For this review, take the finished solid that the model builds, in its own axes (mm). A direction names the side the tool comes from. Coordinates: 2 decimals unless noted, no trailing zeros. Loops run counter-clockwise (first coordinate to the right, second up) from the corner with the lowest first, then second, coordinate; pieces in that order, holes last. Notation, with made-up numbers: M -37.5,62 L 10.5,62 A28 ccw 10.5,88 Z; hole C 11.5,-14.75 d2. An arc over 180 degrees is marked long. Answer as a JSON object with one key per item and string values. Group by question number.
Item 1: Add section B-B (y = 13). State the section outline as (x, z) points, then the cut area to 3 significant figures.
Item 2: Wall thickness on L1, parallel to Y at x = 2, z = -13; L2, parallel to Y at x = -6.5, z = -2.5; L3, parallel to Z at x = 19, y = 13: over which ranges is each line inside the solid? List them lowest first. Write a range as from..to.
Item 3: Mouldability with a two-part tool opening along Z and no side actions: class faces 4 (the face through (1, 0, 0)), 5 (the face through (1, 20, -8)), 6 (the face through (1, 11, -12)) as +Z half, -Z half, draft (parallel to the pull), parting line (faces both ways), or undercut.
Item 4: Add section D-D (y = 0). State the section outline as (x, z) points.
Item 5: Add section C-C (z = -8.75). State the section outline as (x, y) points, then the cut area to 3 significant figures.
Item 6: Insertion check: pin 1 (9 mm diameter, centred on x = 35, y = 0, fed in from -Z); pin 2 (2 mm diameter, centred on y = 11, z = -10.5, fed in from -X). Each pin has a flat end and moves straight along its axis. Give the tip position at first contact, or say it passes through.
Item 7: Tool access review of faces 1 (the face through (1, 15, -15)), 2 (the face through (1, -14, -14)), 3 (the face through (1, 10, -12)): name each direction out of +Z, -Z, +X, -X, +Y, -Y from which nothing blocks a thin tool from reaching the whole face with its end or side.
from build123d import *

# Parameters (mm, degrees)
F1_DEPTH = 52
F2_R     = 4
F3_DEPTH = 12.5
F4_R     = 1
F5_R     = 1
F6_R     = 1


with BuildPart() as f1:
    # F0 (on Right) → F1 (new body, symmetric)
    with BuildSketch(Plane.YZ):
        Polygon((20, 0), (-20, 0), (-20, -15), (-10, -15), (-10, -11), (-11, -11), (-11, -14), (-19, -14), (-19, -1), (19, -1), (19, -14), (11, -14), (11, -11), (10, -11), (10, -15), (20, -15), align=None)
    extrude(amount=F1_DEPTH, both=True)

    # F2 (on Top) → F3 (cut, symmetric)
    with BuildSketch(Plane.XY):
        with Locations((-35, 0)):
            Circle(F2_R)
        with Locations((35, 0)):
            Circle(F2_R)
    extrude(amount=F3_DEPTH, both=True, mode=Mode.SUBTRACT)

    # F4
    f4_edges = [f1.edges().sort_by_distance(p)[0] for p in [
        (0, -20, -15),
        (0, -20, 0),
        (0, -10, -15),
        (0, 10, -15),
        (0, 20, -15),
        (0, 20, 0),
        (0, 19, -14),
        (0, -19, -14),
    ]]
    fillet(f4_edges, radius=F4_R)

    # F5
    f5_edges = [f1.edges().sort_by_distance(p)[0] for p in [
        (0, 11, -14),
        (0, 19, -1),
        (0, -19, -1),
    ]]
    fillet(f5_edges, radius=F5_R)

    # F6
    f6_edges = [f1.edges().sort_by_distance(p)[0] for p in [
        (52, -10.5, -11),
        (52, 10.5, -11),
        (-52, 10.5, -11),
        (-52, -10.5, -11),
    ]]
    fillet(f6_edges, radius=F6_R)


solid = f1.part
From the geometry:
{
 "1": {"outline": "M -52,-15 L 52,-15 L 52,-14 L -52,-14 Z; M -52,-1 L 52,-1 L 52,0 L -52,0 Z", "area": "208 mm²"},
 "2": {"L1": "y = -20..-19, -11..-10, 10..11, 19..20", "L2": "y = -20..-19, 19..20", "L3": "z = -15..-14, -1..0"},
 "3": {"face 4": "+Z half", "face 5": "draft", "face 6": "undercut"},
 "4": {"outline": "M -52,-1 L -39,-1 L -39,0 L -52,0 Z; M -31,-1 L 31,-1 L 31,0 L -31,0 Z; M 39,-1 L 52,-1 L 52,0 L 39,0 Z"},
 "5": {"outline": "M -52,-20 L 52,-20 L 52,-19 L -52,-19 Z; M -52,19 L 52,19 L 52,20 L -52,20 Z", "area": "208 mm²"},
 "6": {"pin 1": "stops at z = -1", "pin 2": "stops at x = -51.87"},
 "7": {"face 1": "-Z, +X, -X, +Y, -Y", "face 2": "+X, -X", "face 3": "-Z, +X, -X"}
}
